Input: part model. Units: mm. Frame: model coordinates. Face numbers are marked on the shaded views. A direction names the side the tool comes from. Round coordinates to 2 decimals unless told otherwise and drop trailing zeros. Order: outer loops, then holes, each group sorted by start corner. A loop starts at its lowest first (then second) coordinate and runs counter-clockwise, first axis right, second up.
Item 1: First-contact query: pin 1 (1.2 mm diameter, centred on x = -4.5, z = 1, fed in from +Y); pin 2 (5 mm diameter, centred on x = 9.5, z = 1, fed in from +Y); pin 3 (4.5 mm diameter, centred on x = -26.5, y = -14.5, fed in from +Z); pin 4 (4.5 mm diameter, centred on x = 31, y = 42.08, fed in from -Z). Flat tips, straight axial feed; report the tip coordinate or a pass-through.
Item 2: Cut plane B-B on y = 0. Output: boundary loops of the cut face in (x, z), then the cut area to 3 significant figures.
Item 3: Reachability of the marked faces 1, 2 and 3 from +Z, -Z, +X, -X, +Y, -Y: full face, straight path, thin tool, end or side. Return the list, or none.
Item 4: Cut plane A-A on x = 11.5. Output: boundary loops of the cut face in (y, z), then the cut area to 3 significant figures.
Item 5: Line query: L1, parallel to Y at x = 0, z = -5.35; L2, parallel to Y at x = 19, z = -1.25; L3, parallel to Y at x = 19, z = -3.5. Output: solid intervals per line, ascending.
```python
from build123d import *

# Parameters (mm, degrees)
BOSS_EXTRUDE1_DEPTH        = 2.6
BOSS_EXTRUDE1_DEPTH_BACK   = 6
FILLET1_R                  = 20
CUT_EXTRUDE1_DEPTH         = 5
SKETCH5_R                  = 2
CUT_EXTRUDE2_DEPTH         = 20
FILLET3_R                  = 1
CIRPATTERN1_COUNT          = 3
SKETCH6_R                  = 2.75
CUT_EXTRUDE3_DEPTH         = 56.475677209
BOSS_EXTRUDE2_DEPTH        = 4
SKETCH8_R                  = 2.1
CUT_EXTRUDE4_DEPTH         = 85.036841694
CHAMFER1_SIZE              = 2.5
SKETCH9_R                  = 1.5
CUT_EXTRUDE5_DEPTH         = 85.036841694
BOSS_EXTRUDE3_DEPTH        = 5.2
BOSS_EXTRUDE4_DEPTH        = 5.2
FILLET4_R                  = 10
SKETCH13_R                 = 7
CUT_EXTRUDE7_DEPTH         = 5
SKETCH14_W                 = 50
SKETCH14_H                 = 35.2
CUT_EXTRUDE8_DEPTH         = 1.2
F_5_6_5_6_DIAMETER_HOLE1_D = 5.6
SKETCH17_R                 = 12.75
CUT_EXTRUDE9_DEPTH         = 85.036841694


with BuildPart() as part:
    # Sketch3 → Boss-Extrude1 (new, two sides: drawn at the far end of the back side and taken through both)
    with BuildSketch(Plane.XY.offset(-BOSS_EXTRUDE1_DEPTH_BACK)):
        Polygon((-25, 39), (25, 39), (25, -3.511595657), (38.504425224, -11.308379196), (33.774990748, -19.5), (29.045556271, -27.691620804), (-29.045556271, -27.691620804), (-33.774990748, -19.5), (-38.504425224, -11.308379196), (-25, -3.511595657), align=None)
    extrude(amount=BOSS_EXTRUDE1_DEPTH + BOSS_EXTRUDE1_DEPTH_BACK)

    # Fillet1
    fillet1_edges = [part.edges().sort_by_distance(p)[0] for p in [
        (25, -3.511595657, -1.7),
        (-25, -3.511595657, -1.7),
    ]]
    fillet(fillet1_edges, radius=FILLET1_R)

    # Sketch4 → Cut-Extrude1 (cut, symmetric)
    with BuildSketch(Plane(origin=(0, 30, 0), x_dir=(1, 0, 0), z_dir=(0, 1, 0))):
        Polygon((5.114783638, 0.485216362), (-5.114783638, 0.485216362), (-6, -0.4), (-6, -2.6), (6, -2.6), (6, -0.4), align=None)
    cut_extrude1 = extrude(amount=CUT_EXTRUDE1_DEPTH, both=True, mode=Mode.SUBTRACT)

    # Sketch5 → Cut-Extrude2 (cut)
    with BuildSketch(Plane(origin=(0, 39, 0), x_dir=(1, 0, 0), z_dir=(0, 1, 0))):
        with Locations(Location((-4.458868953, 0, 0), (0, 0, 180))):
            Circle(SKETCH5_R)
        with Locations(Location((4.458868953, 0, 0), (0, 0, 180))):
            Circle(SKETCH5_R)
    cut_extrude2 = extrude(amount=-CUT_EXTRUDE2_DEPTH, mode=Mode.SUBTRACT)

    # Fillet3
    fillet3_edges = [part.edges().sort_by_distance(p)[0] for p in [
        (-6, 30, 2.6),
        (6, 30, 2.6),
    ]]
    fillet(fillet3_edges, radius=FILLET3_R)

    # CirPattern1: Cut-Extrude1, Cut-Extrude2 ×3 about axis
    cirpattern1_axis = Axis((0, 0, 0), (0, 0, 1))
    add([cut_extrude1.rotate(cirpattern1_axis, i * 360 / CIRPATTERN1_COUNT) for i in range(1, CIRPATTERN1_COUNT)], mode=Mode.SUBTRACT)
    add([cut_extrude2.rotate(cirpattern1_axis, i * 360 / CIRPATTERN1_COUNT) for i in range(1, CIRPATTERN1_COUNT)], mode=Mode.SUBTRACT)

    # Sketch6 → Cut-Extrude3 (cut, through all)
    with BuildSketch(Plane.XY.offset(2.6)):
        Circle(SKETCH6_R)
    extrude(amount=-CUT_EXTRUDE3_DEPTH, mode=Mode.SUBTRACT)

    # Sketch7 → Boss-Extrude2 (add)
    with BuildSketch(Plane(origin=(0, 0, -6), x_dir=(-1, 0, 0), z_dir=(0, 0, -1))):
        with BuildLine():
            Line((-25, 39), (25, 39))
            Line((25, 39), (25, 54))
            Line((25, 54), (3.986839478, 72.68387232))
            ThreePointArc((3.986839478, 72.68387232), (0, 74.2), (-3.986839478, 72.68387232))
            Line((-3.986839478, 72.68387232), (-25, 54))
            Line((-25, 54), (-25, 39))
        make_face()
    extrude(amount=-BOSS_EXTRUDE2_DEPTH)

    # Sketch8 → Cut-Extrude4 (cut, through all)
    with BuildSketch(Plane.XY.offset(2.6)):
        with Locations((-19, 15.7)):
            Circle(SKETCH8_R)
        with Locations((19, 15.7)):
            Circle(SKETCH8_R)
        with Locations((0, 68.2)):
            Circle(SKETCH8_R)
    extrude(amount=-CUT_EXTRUDE4_DEPTH, mode=Mode.SUBTRACT)

    # Chamfer1
    chamfer1_edges = [part.edges().sort_by_distance(p)[0] for p in [
        (-21.1, 15.7, 2.6),
        (16.9, 15.7, 2.6),
        (-2.1, 68.2, -2),
    ]]
    chamfer(chamfer1_edges, length=CHAMFER1_SIZE)

    # Sketch9 → Cut-Extrude5 (cut, through all)
    with BuildSketch(Plane(origin=(0, 0, -6), x_dir=(-1, 0, 0), z_dir=(0, 0, -1))):
        with Locations((7.5, -21.041620804)):
            Circle(SKETCH9_R)
        with Locations((-2, -21.041620804)):
            Circle(SKETCH9_R)
    extrude(amount=-CUT_EXTRUDE5_DEPTH, mode=Mode.SUBTRACT)

    # Sketch10 → Boss-Extrude3 (add)
    with BuildSketch(Plane(origin=(0, 0, -6), x_dir=(-1, 0, 0), z_dir=(0, 0, -1))):
        with BuildLine():
            Line((25, 8.035409726), (25, 54))
            Line((25, 54), (3.986839478, 72.68387232))
            ThreePointArc((3.986839478, 72.68387232), (2.132693846, 73.80817412), (0, 74.2))
            Line((0, 74.2), (38.504425224, 74.2))
            Line((38.504425224, 74.2), (38.504425224, -11.308379196))
            Line((38.504425224, -11.308379196), (35, -9.285098349))
            ThreePointArc((35, -9.285098349), (27.679491924, -1.964590274), (25, 8.035409726))
        make_face()
    extrude(amount=-BOSS_EXTRUDE3_DEPTH)

    # Sketch11 → Boss-Extrude4 (add)
    with BuildSketch(Plane(origin=(0, 0, -6), x_dir=(-1, 0, 0), z_dir=(0, 0, -1))):
        with BuildLine():
            Line((-38.504425224, -11.308379196), (-38.504425224, 74.2))
            Line((-38.504425224, 74.2), (0.121007206, 74.2))
            Line((0.121007206, 74.2), (-25, 54))
            Line((-25, 54), (-25, 8.035409726))
            ThreePointArc((-25, 8.035409726), (-27.679491924, -1.964590274), (-35, -9.285098349))
            Line((-35, -9.285098349), (-38.504425224, -11.308379196))
        make_face()
    extrude(amount=-BOSS_EXTRUDE4_DEPTH)

    # Fillet4
    fillet4_edges = [part.edges().sort_by_distance(p)[0] for p in [
        (-38.504425224, 74.2, -3.4),
        (38.504425224, 74.2, -3.4),
    ]]
    fillet(fillet4_edges, radius=FILLET4_R)

    # Sketch13 → Cut-Extrude7 (cut)
    with BuildSketch(Plane(origin=(0, 0, -6), x_dir=(-1, 0, 0), z_dir=(0, 0, -1))):
        Circle(SKETCH13_R)
    extrude(amount=-CUT_EXTRUDE7_DEPTH, mode=Mode.SUBTRACT)

    # Sketch14 → Cut-Extrude8 (cut)
    with BuildSketch(Plane.XY.offset(-0.8)):
        with Locations((0, 56.6)):
            Rectangle(SKETCH14_W, SKETCH14_H)
    extrude(amount=-CUT_EXTRUDE8_DEPTH, mode=Mode.SUBTRACT)

    # Ø5.6 (5.6) Diameter Hole1 (through all)
    with Locations(Plane.XY.offset(-0.8)):
        with Locations((-31, 49.8275), (-31, 31.0775), (31, 42.0775), (31, 60.8275)):
            Hole(F_5_6_5_6_DIAMETER_HOLE1_D / 2)

    # Sketch17 → Cut-Extrude9 (cut, through all)
    with BuildSketch(Plane(origin=(0, 0, -6), x_dir=(-1, 0, 0), z_dir=(0, 0, -1))):
        Circle(SKETCH17_R)
    extrude(amount=-CUT_EXTRUDE9_DEPTH, mode=Mode.SUBTRACT)


solid = part.part
```
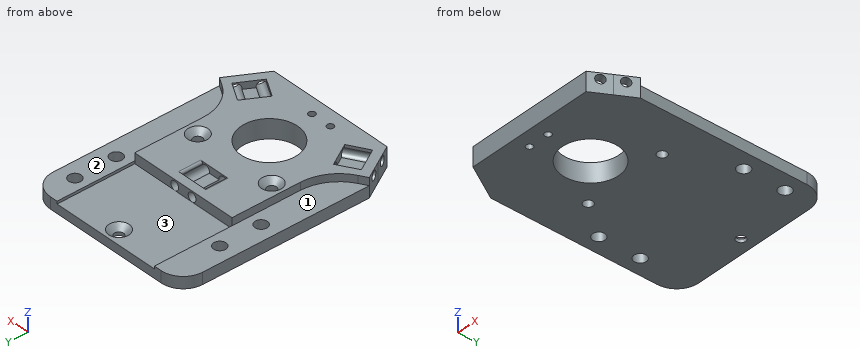
From the geometry:
1. pin 1: stops at y = 19
1. pin 2: stops at y = 39
1. pin 3: stops at z = -0.49
1. pin 4: passes through
2. outline: (-38.5, -6) - (-12.75, -6) - (-12.75, 2.6) - (-26.69, 2.6) - (-26.69, -0.8) - (-38.5, -0.8) - close; (12.75, -6) - (38.5, -6) - (38.5, -0.8) - (26.69, -0.8) - (26.69, 2.6) - (12.75, 2.6) - close
2. area: 363 mm2
3. face 1: +Z, -X, +Y
3. face 2: +Z, +X, +Y
3. face 3: +Z, +Y
4. outline: (-27.69, -6) - (-5.51, -6) - (-5.51, 2.6) - (-27.69, 2.6) - close; (5.51, -6) - (74.2, -6) - (74.2, -2) - (39, -2) - (39, 2.6) - (5.51, 2.6) - close
4. area: 620 mm2
5. L1: y = -27.69 to -12.75, 12.75 to 66.1, 70.3 to 74.2
5. L2: y = -27.69 to -17.92, -14.32 to -7.62, -5.09 to 13.6, 17.8 to 39
5. L3: y = -27.69 to 13.6, 17.8 to 74.2
